from build123d import *

# Parameters (mm, degrees)
BOSS_EXTRUDE1_DEPTH = 12
SKETCH2_R           = 3.5
CUT_EXTRUDE1_DEPTH  = 1
SKETCH3_R           = 1.55
CUT_EXTRUDE2_DEPTH  = 3.1
SKETCH5_R           = 1.55
CUT_EXTRUDE3_DEPTH  = 11


with BuildPart() as part:
    # Sketch1 → Boss-Extrude1 (new body)
    with BuildSketch(Plane.XY):
        Polygon((0, 13.037037037), (-3, 13.037037037), (-3, -13.962962963), (15, -13.962962963), (15, -11.962962963), (0, -11.962962963), align=None)
    extrude(amount=BOSS_EXTRUDE1_DEPTH)

    # Sketch2 → Cut-Extrude1 (cut)
    with BuildSketch(Plane.ZY.offset(3)):
        with Locations(Location((6.055399975, -9.462962963, 0), (0, 0, 270))):
            Circle(SKETCH2_R)
        with Locations(Location((6.276999876, 8.537037037, 0), (0, 0, 270))):
            Circle(SKETCH2_R)
    extrude(amount=-CUT_EXTRUDE1_DEPTH, mode=Mode.SUBTRACT)

    # Sketch3 → Cut-Extrude2 (cut)
    with BuildSketch(Plane.ZY.offset(3)):
        with Locations(Location((6.276999876, 8.537037037, 0), (0, 0, 270))):
            Circle(SKETCH3_R)
    extrude(amount=-CUT_EXTRUDE2_DEPTH, mode=Mode.SUBTRACT)

    # Sketch5 → Cut-Extrude3 (cut)
    with BuildSketch(Plane(origin=(0, 0, 0), x_dir=(0, 0, -1), z_dir=(1, 0, 0))):
        with Locations(Location((-6, -9.462962963, 0), (0, 0, 90))):
            Circle(SKETCH5_R)
    extrude(amount=-CUT_EXTRUDE3_DEPTH, mode=Mode.SUBTRACT)


solid = part.part
Geometry check sheet. Reference: the model listing, model coordinates, mm. A direction names the side the tool comes from. Give positions to 0.01 mm unless a question says otherwise; leave off trailing zeros. Write each loop counter-clockwise with the first axis right and the second up, starting at its lowest first coordinate (ties: lowest second). Pieces come first, ordered by that corner, then holes.
1) Cross-section at C-C (x = -0.5). Record the boundary of the cut face in (y, z).
Values follow:
outline: (-13.96, 0) - (13.04, 0) - (13.04, 12) - (-13.96, 12) - close; hole circle Ø3.1 at (-9.46, 6); hole circle Ø3.1 at (8.54, 6.28)
2) Cross-section at D-D (y = 6.5). Record the boundary of the cut face in (x, z).
Values follow:
outline: (-3, 0) - (0, 0) - (0, 12) - (-3, 12) - (-3, 9.12) - (-2, 9.12) - (-2, 3.43) - (-3, 3.43) - close
3) Release check for a two-part mould opening along Y. For faces 1 (the face through (8, -11.963, 6)), 2 (the face through (15, -13, 6)), 3 (the face through (-2.507, -6.685, 3.926)) record: released by +Y, released by -Y, zero draft, split by the parting line, or undercut.
Values follow:
face 1: released by +Y
face 2: zero draft
face 3: undercut
4) Cross-section at B-B (z = 1.5). Record the boundary of the cut face in (x, y).
Values follow:
outline: (-3, -13.96) - (15, -13.96) - (15, -11.96) - (0, -11.96) - (0, 13.04) - (-3, 13.04) - close
5) Thickness scan on line 1 (Y direction, x = 8.25, z = 7); line 2 (X direction, y = -2, z = 0.5); line 3 (Y direction, x = -1.5, z = 5.25). Record the ranges inside material, lowest first.
Values follow:
line 1: y = -13.96 to -11.96
line 2: x = -3 to 0
line 3: y = -13.96 to -10.82, -8.11 to 7.38, 9.7 to 13.04
6) Cross-section at A-A (y = 9.25). Record the boundary of the cut face in (x, z), plus the area to 3 significant figures.
Values follow:
outline: (-3, 0) - (0, 0) - (0, 4.9) - (-2, 4.9) - (-2, 2.85) - (-3, 2.85) - close; (-3, 9.7) - (-2, 9.7) - (-2, 7.65) - (0, 7.65) - (0, 12) - (-3, 12) - close
area: 23.6 mm2
7) Set-up check for faces 4 (the face through (-0.986, -8.63, 7.307)), 5 (the face through (0, 0, 6)), 6 (the face through (-2.507, 12.034, 6.431)): record each of +Z, -Z, +X, -X, +Y, -Y from which the full face is reachable in a straight line by a thin tool's end or side.
Values follow:
face 4: +X, -X
face 5: +Z, -Z, +X, +Y
face 6: -X
8) Go/stop test with flat-tipped pins: pin 1 Ø1 at (x, z) = (7, 1.5) entering from +Y; pin 2 Ø1.5 at (y, z) = (-9.5, 2.5) entering from +X; pin 3 Ø5.5 at (y, z) = (-9.46, 6.06) entering from -X. Record where each tip stops, or that it passes through.
Values follow:
pin 1: stops at y = -11.96
pin 2: stops at x = 0
pin 3: stops at x = -2
